Autodesk Inventor part; units mm, degrees
ref_plane "Work Plane1" through (42.5, 55, 0) normal (0, 0.8660254, -0.5) x (-1, 0, 0)
ref_plane "YZ Plane" through (0, 0, 0) normal (1, 0, 0) x (0, 1, 0)
ref_plane "XZ Plane" through (0, 0, 0) normal (0, 1, 0) x (-1, 0, 0)
sketch "Sketch1" plane through (0, 0, 0) normal (0, 0, 1) x (1, 0, 0)
  circle A0 centre (0, 0) radius 5
  circle A1 centre (65, 0) radius 5
  circle A2 centre (0, 0) radius 12.5
  circle A3 centre (65, 0) radius 12.5
  line L0 (22.5, 9.5) -> (42.5, 9.5)
  line L1 (42.5, 9.5) -> (42.5, -10.5)
  line L2 (42.5, -10.5) -> (22.5, -10.5)
  line L3 (22.5, -10.5) -> (22.5, 9.5)
  line L4 (0, 0) -> (65, 0) construction
  line L5 (32.5, 0) -> (32.5, 30) construction
  line L6 (27.5, 30) -> (37.5, 30)
  line L7 (12.5, 0) -> (12.5, 15)
  line L8 (52.5, 0) -> (52.5, 15)
  arc A4 (27.5, 30) -> (12.5, 15) centre (27.5, 15) ccw
  arc A5 (52.5, 15) -> (37.5, 30) centre (37.5, 15) ccw
  line L9 (-12.5, 0) -> (-12.5, 20)
  line L10 (77.5, 0) -> (77.5, 20)
  line L11 (22.5, 55) -> (42.5, 55)
  arc A6 (22.5, 55) -> (-12.5, 20) centre (22.5, 20) ccw
  arc A7 (77.5, 20) -> (42.5, 55) centre (42.5, 20) ccw
  point P0 (22.5, 30)
  point P1 (42.5, 30)
  dimension "d0" = 10
  dimension "d1" = 10
  dimension "d2" = 65
  dimension "d3" = 25
  dimension "d4" = 25
  dimension "d5" = 22.5
  dimension "d6" = 22.5
  dimension "d7" = 9.5
  dimension "d8" = 10.5
  dimension "d11" = 20
  dimension "d12" = 10
  dimension "d13" = 30
  dimension "d14" = 15
  dimension "d15" = 55
  dimension "d16" = 35
extrude "Extrusion1" add sketch "Sketch1" along normal blind 30 contours A2 | A2 L9 A6 L11 A7 L10 A3 L8 A5 L6 A4 L7 | A3
ref_plane "Work Plane1" through (42.5, 55, 0) normal (0, 0.8660254, -0.5) x (-1, 0, 0)
sketch "Sketch2" plane through (42.5, 55, 0) normal (0, 0.8660254, -0.5) x (-1, 0, 0)
  line L0 (0, 0) -> (20, 0)
  line L1 (20, 0) -> (20, 25.9808)
  line L2 (0, 25.9808) -> (20, 25.9808)
  line L3 (0, 0) -> (0, 25.9808)
  line L4 (15, -12.5) -> (5, -12.5)
  line L5 (5, -12.5) -> (5, 13.4808)
  line L6 (15, 13.4808) -> (5, 13.4808)
  line L7 (15, -12.5) -> (15, 13.4808)
  circle A0 centre (10, 6.7404) radius 5
  circle A1 centre (10, 6.7404) radius 12.5
  point P0 (42.5, -27.5)
  dimension "d20" = 38.4808
  dimension "d21" = 19.2404
  dimension "d22" = 20
  dimension "d23" = 10
  dimension "d24" = 10
  dimension "d25" = 25
extrude "Extrusion6" cut sketch "Sketch2" against normal blind 55.75 contours A0
extrude "Extrusion7" add sketch "Sketch2" against normal blind 39.25 contours L3 A1 L1 L0 L7 L6 L5 | L0 L5 A1 L3 | L5 A0 L7 L0 | L0 L7 A1 L5 | L0 L1 A1 L7 | L5 L6 L7 A0
sketch "Sketch5" plane through (32.5, 24.3787, 25.4623) normal (0, -0.8660254, 0.5) x (-1, 0, 0)
  circle A0 centre (0, 0) radius 5
  circle A1 centre (0, 0) radius 12.5
  point P0 (32.5, 34.2404)
extrude "Extrusion8" cut sketch "Sketch5" against normal blind 6
sketch "Sketch6" plane through (22.5, 55, 30) normal (0, 1, 0) x (1, 0, 0)
  ellipse E0 centre (10, 7.5377) end of major axis (22.5, 7.5377) minor radius 10.8253 (1.0281, 0) -> (18.9719, 0) ccw
  line L0 (1.0281, 0) -> (18.9719, 0)
  point P0 (-22.5, 30)
extrude "Extrusion9" cut sketch "Sketch6" against normal blind 41
fillet "Fillet3" radius 1.5 2 edges at (20.4586, 31.2539, 25.3665) (44.5414, 31.2539, 25.3665)
equation "\"d15\" = d13 + d3"
equation "\"d21\" = 0.5 * d20"
equation "\"d23\" = 0.5 * d22"
properties part number "Mount"
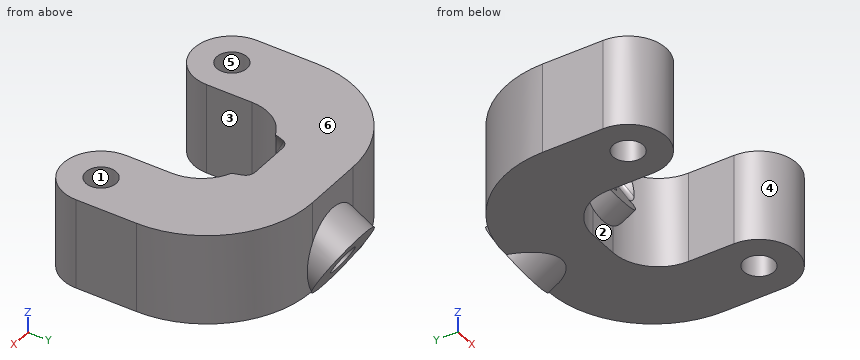
For this review, take the finished solid that the model builds, in its own axes (mm). Face numbers are marked on the shaded views. A direction names the side the tool comes from. Give positions to 0.01 mm unless a question says otherwise; leave off trailing zeros. Loops run counter-clockwise (first coordinate to the right, second up) from the corner with the lowest first, then second, coordinate; pieces in that order, holes last. Notation, with made-up numbers: M 6.25,28 L 47.25,28 A9 cw 47.25,39 Z; hole C 62,8 d9. An arc over 180 degrees is marked long. Answer as a JSON object with one key per item and string values. Group by question number.
Q1. Add section C-C on x = 54. Give the boundary of the cut face in (y, z).
Q2. Tool access review of the marked faces 1, 2 and 3: name each direction out of +Z, -Z, +X, -X, +Y, -Y from which nothing blocks a thin tool from reaching the whole face with its end or side.
Q3. Add section D-D on x = 0. Give the boundary of the cut face in (y, z).
Q4. Mouldability with a two-part tool opening along Y and no side actions: class the marked faces 4, 5 and 6 as +Y half, -Y half, draft (parallel to the pull), parting line (faces both ways), or undercut.
Q5. For probe 1 along X at (y, z) = (14.5, 25.5); probe 2 along Z at (x, y) = (18.5, 46); probe 3 along Y at (x, z) = (65, 22.25), list the stretches that pass through material, from the lowest coordinate up. Write a range as [from, to].
Q6. Add section B-B on x = 67.5. Give the boundary of the cut face in (y, z), and give its area (3 significant figures).
Q7. Add section A-A on y = 2. Give the boundary of the cut face in (x, z), and give its area (3 significant figures).
Q8. Insertion check: P1, Ø1.5, axis at y = 51.5, z = 6, coming from the -X side; P2, Ø1.5, axis at x = 30, z = 1.5, coming from the -Y side; P3, Ø8, axis at x = 32.5, z = 8.5, coming from the +Y side. Each pin has a flat end and moves straight along its axis. Give the tip position at first contact, or say it passes through.
Checked values:
{
 "1": {"outline": "M -5.94,0 L 53.06,0 L 53.06,30 L -5.94,30 Z"},
 "2": {"face 1": "+Z, -Z", "face 2": "-Z, -Y", "face 3": "+Z, -Z, -Y"},
 "3": {"outline": "M -12.5,0 L -5,0 L -5,30 L -12.5,30 Z; M 5,0 L 46.81,0 L 46.81,30 L 5,30 Z"},
 "4": {"face 4": "-Y half", "face 5": "undercut", "face 6": "draft"},
 "5": {"probe 1": "[-12.5, 12.5], [52.5, 77.5]", "probe 2": "[0, 30]", "probe 3": "[-12.5, -5], [5, 46.81]"},
 "6": {"outline": "M -12.25,0 L -4.33,0 L -4.33,30 L -12.25,30 Z; M 4.33,0 L 44.49,0 L 44.49,30 L 4.33,30 Z", "area": "1,440 mm²"},
 "7": {"outline": "M -12.5,0 L -4.58,0 L -4.58,30 L -12.5,30 Z; M 4.58,0 L 12.5,0 L 12.5,30 L 4.58,30 Z; M 52.5,0 L 60.42,0 L 60.42,30 L 52.5,30 Z; M 69.58,0 L 77.5,0 L 77.5,30 L 69.58,30 Z", "area": "950 mm²"},
 "8": {"P1": "x = 5.78", "P2": "y = 30", "P3": "y = 62.22"}
}
